from build123d import *

# Parameters (mm, degrees)
BOSS_EXTRUDE1_DEPTH = 3


with BuildPart() as part:
    # Sketch1 → Boss-Extrude1 (new body)
    with BuildSketch(Plane(origin=(0, 0, 0), x_dir=(1, 0, 0), z_dir=(0, 1, 0))):
        with BuildLine():
            Line((4.475348529, 54.140378085), (9.517238433, 6.17))
            Line((9.517238433, 6.17), (12.686230549, 6.513661021))
            ThreePointArc((12.686230549, 6.513661021), (14.15792829, 6.081687043), (14.890899928, 4.734375521))
            Line((14.890899928, 4.734375521), (15.538277417, -1.425009852))
            ThreePointArc((15.538277417, -1.425009852), (17.186852955, -2.76), (18.521843103, -1.111424462))
            Line((18.521843103, -1.111424462), (17.283321421, 10.672322207))
            Line((17.283321421, 10.672322207), (18.076495252, 10.884852494))
            ThreePointArc((18.076495252, 10.884852494), (22.84818786, 9.935703821), (25, 5.572260449))
            Line((25, 5.572260449), (25, 0.469626618))
            ThreePointArc((25, 0.469626618), (24.758369054, -4.440028067), (24.035811635, -9.302229772))
            Line((24.035811635, -9.302229772), (23.801666433, -10.477185639))
            ThreePointArc((23.801666433, -10.477185639), (22.069368276, -13.36561303), (18.89808527, -14.5))
            Line((18.89808527, -14.5), (12.85, -14.5))
            Line((12.85, -14.5), (12.85, -10.55))
            ThreePointArc((12.85, -10.55), (9.28, -6.98), (5.71, -10.55))
            Line((5.71, -10.55), (5.71, -14.5))
            Line((5.71, -14.5), (1.5, -14.5))
            Line((1.5, -14.5), (1.5, 0))
            ThreePointArc((1.5, 0), (0, 1.5), (-1.5, 0))
            Line((-1.5, 0), (-1.5, -14.5))
            Line((-1.5, -14.5), (-5.71, -14.5))
            Line((-5.71, -14.5), (-5.71, -10.55))
            ThreePointArc((-5.71, -10.55), (-9.28, -6.98), (-12.85, -10.55))
            Line((-12.85, -10.55), (-12.85, -14.5))
            Line((-12.85, -14.5), (-18.89808527, -14.5))
            ThreePointArc((-18.89808527, -14.5), (-22.069368276, -13.36561303), (-23.801666433, -10.477185639))
            Line((-23.801666433, -10.477185639), (-24.035811635, -9.302229772))
            ThreePointArc((-24.035811635, -9.302229772), (-24.758369054, -4.440028067), (-25, 0.469626618))
            Line((-25, 0.469626618), (-25, 5.572260449))
            ThreePointArc((-25, 5.572260449), (-22.84818786, 9.935703821), (-18.076495252, 10.884852494))
            Line((-18.076495252, 10.884852494), (-17.283321421, 10.672322207))
            Line((-17.283321421, 10.672322207), (-18.521843103, -1.111424462))
            ThreePointArc((-18.521843103, -1.111424462), (-17.186852955, -2.76), (-15.538277417, -1.425009852))
            Line((-15.538277417, -1.425009852), (-14.890899928, 4.734375521))
            ThreePointArc((-14.890899928, 4.734375521), (-14.15792829, 6.081687043), (-12.686230549, 6.513661021))
            Line((-12.686230549, 6.513661021), (-9.517238433, 6.17))
            Line((-9.517238433, 6.17), (-4.475348529, 54.140378085))
            ThreePointArc((-4.475348529, 54.140378085), (0, 58.17), (4.475348529, 54.140378085))
        make_face()
    extrude(amount=BOSS_EXTRUDE1_DEPTH)


solid = part.part
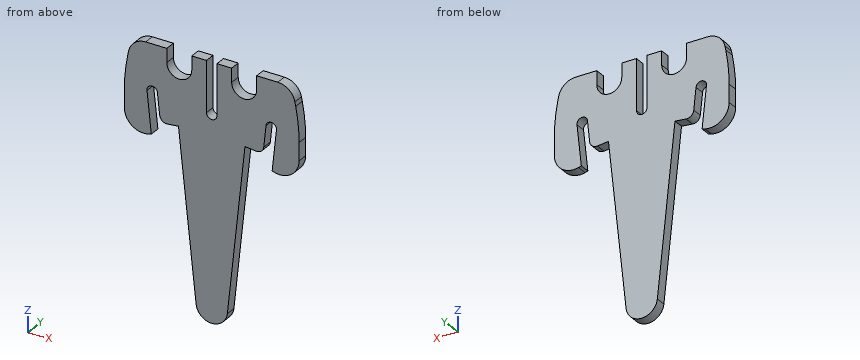
Can you work these out from the model? Positions are in its coordinate system, mm. Coordinates: 2 decimals unless noted, no trailing zeros. Order: outer loops, then holes, each group sorted by start corner. A loop starts at its lowest first (then second) coordinate and runs counter-clockwise, first axis right, second up. Notation, with made-up numbers: (-35, 42) - (-15, 42) arc R23 ccw to (-15, 74) - close; hole circle Ø10 at (-5.75, 33.5). An arc over 180 degrees is marked (long way). Answer as a JSON object with one key per item and string values. Group by question number.
Q1. Will these pins go through, and if not, where does the flat tip stop? P1, Ø0.9, axis at y = 1.5, z = 10, coming from the -X side; P2, Ø5, axis at x = 9.5, z = -46.5, coming from the -Y side.
Q2. Imagine slicing it at B-B (x = 0). Please give me the cut outline in (y, z), and give its area (3 significant figures).
Q3. Imagine slicing it at A-A (z = -21). Please give me the cut outline in (x, y).
Q4. I need wall thicknesses on line 1 (X direction, y = 1.25, z = -2.5); line 2 (X direction, y = 0.2, z = 11); line 3 (X direction, y = 1.8, z = 9). Which ranges of each line are inside material? Lowest first, please. Write a range as from..to.
Determined:
{
 "1": {"P1": "stops at x = -23.99", "P2": "passes through"},
 "2": {"outline": "(0, -58.17) - (3, -58.17) - (3, -1.5) - (0, -1.5) - close", "area": "170 mm2"},
 "3": {"outline": "(-7.96, 0) - (7.96, 0) - (7.96, 3) - (-7.96, 3) - close"},
 "4": {"line 1": "x = -25..-18.14, -15.13..15.13, 18.14..25", "line 2": "x = -23.67..-12.85, -5.71..-1.5, 1.5..5.71, 12.85..23.67", "line 3": "x = -24.1..-12.5, -6.06..-1.5, 1.5..6.06, 12.5..24.1"}
}
